Autodesk Inventor part; units mm, degrees
ref_plane "YZ Plane" through (0, 0, 0) normal (1, 0, 0) x (0, 1, 0)
ref_plane "XZ Plane" through (0, 0, 0) normal (0, 1, 0) x (-1, 0, 0)
ref_plane "XY Plane" through (0, 0, 0) normal (0, 0, 1) x (1, 0, 0)
sketch "スケッチ1" plane through (0, 0, 0) normal (0, 0, 1) x (1, 0, 0)
  line L0 (-9.75, -19.5) -> (9.75, -19.5) construction
  line L1 (9.75, -19.5) -> (9.75, 19.5) construction
  line L2 (9.75, 19.5) -> (-9.75, 19.5) construction
  line L3 (-9.75, 19.5) -> (-9.75, -19.5) construction
  line L4 (-9.75, -19.5) -> (9.75, 19.5) construction
  line L5 (9.75, -19.5) -> (-9.75, 19.5) construction
  line L6 (-9.75, 10.5) -> (-9.75, 19.5) construction
  line L7 (-9.75, 19.5) -> (9.75, 19.5)
  line L8 (9.75, 19.5) -> (9.75, 10.5) construction
  line L9 (-9.75, 10.5) -> (-11.75, 10.5)
  line L10 (-11.75, 10.5) -> (-11.75, -10.5)
  line L11 (-11.75, -10.5) -> (-9.75, -10.5)
  line L12 (-9.75, -10.5) -> (-9.75, -19.5) construction
  line L13 (-9.75, -19.5) -> (9.75, -19.5)
  line L14 (9.75, -19.5) -> (9.75, -10.5) construction
  line L15 (9.75, -10.5) -> (12.75, -10.5)
  line L16 (12.75, -10.5) -> (12.75, 10.5)
  line L17 (12.75, 10.5) -> (9.75, 10.5)
  line L18 (0, 0) -> (12.75, 0) construction
  circle A0 centre (-9.75, 11.55) radius 1.05 construction
  circle A1 centre (-9.75, -11.55) radius 1.05 construction
  circle A2 centre (9.75, 11.55) radius 1.05 construction
  circle A3 centre (9.75, -11.55) radius 1.05 construction
  line L19 (-9.75, 19.5) -> (-9.75, 12.6)
  arc A4 (-9.75, 10.5) -> (-9.75, 12.6) centre (-9.75, 11.55) ccw
  arc A5 (-9.75, -12.6) -> (-9.75, -10.5) centre (-9.75, -11.55) ccw
  line L20 (-9.75, -12.6) -> (-9.75, -19.5)
  line L21 (9.75, 12.6) -> (9.75, 19.5)
  arc A6 (9.75, 12.6) -> (9.75, 10.5) centre (9.75, 11.55) ccw
  line L22 (9.75, -12.6) -> (9.75, -19.5)
  arc A7 (9.75, -10.5) -> (9.75, -12.6) centre (9.75, -11.55) ccw
  dimension "d21" = 2
  dimension "d23" = 3
  dimension "d30" = 19.5
  dimension "d48" = 9
  dimension "d49" = 39
  dimension "d50" = 2.1
extrude "押し出し1" add sketch "スケッチ1" along normal blind 5
sketch "スケッチ2" plane through (9.75, -19.5, 0) normal (1, 0, 0) x (0, 0, -1)
  line L0 (0, 0) -> (-5, 0)
  line L1 (0, 39) -> (-5, 39)
  point P0 (0, 19.5)
  point P1 (-2.5, 4)
  point P2 (-2.5, 35)
  point P3 (-2.5, 0)
  dimension "d53" = 4
  dimension "d54" = 4
hole "穴1" at (9.75, -15.5, 2.5) at (9.75, 15.5, 2.5) direction (-1, 0, 0) diameter 2.459 depth 2.5 tip angle 118
mirror "ミラー1" about plane through (0, 0, 0) normal (1, 0, 0) of "穴1"
sketch "スケッチ3" plane through (0, 0, 5) normal (0, 0, 1) x (1, 0, 0)
  line L0 (9.75, 12.6) -> (9.75, 19.5)
  line L1 (-9.75, 19.5) -> (-9.75, 12.6)
  line L2 (-14.3307, 15.6684) -> (-9.75, 15.6684)
  line L3 (-9.75, 15.6684) -> (-9.75, -16.7148)
  line L4 (-9.75, -16.7148) -> (-14.3307, -16.7148)
  line L5 (-14.3307, -16.7148) -> (-14.3307, 15.6684)
  line L6 (15.2214, 11.55) -> (9.75, 11.55)
  line L7 (9.75, 11.55) -> (9.75, -15.9078)
  line L8 (9.75, -15.9078) -> (15.2214, -15.9078)
  line L9 (15.2214, -15.9078) -> (15.2214, 11.55)
  point P0 (0, 0)
extrude "押し出し2" cut sketch "スケッチ3" against normal blind 2.5
sketch "スケッチ4" plane through (0, 0, 5) normal (0, 0, 1) x (1, 0, 0)
  line L0 (9.75, 12.6) -> (9.75, 19.5)
  line L1 (9.75, 19.5) -> (-9.75, 19.5)
  line L2 (-9.75, -12.6) -> (-9.75, -19.5)
  line L3 (-9.75, -19.5) -> (9.75, -19.5)
  line L4 (-5.75, 15.5) -> (5.75, 15.5) construction
  line L5 (5.75, 15.5) -> (5.75, -15.5) construction
  line L6 (5.75, -15.5) -> (-5.75, -15.5) construction
  line L7 (-5.75, -15.5) -> (-5.75, 15.5) construction
  line L8 (5.75, 15.5) -> (-5.75, -15.5) construction
  line L9 (3.6168, 15.5) -> (-5.75, 15.5)
  line L10 (-5.75, 15.5) -> (-5.75, -9.7497)
  line L11 (-5.75, -9.7497) -> (3.6168, 15.5)
  line L12 (-3.6168, -15.5) -> (5.75, -15.5)
  line L13 (5.75, -15.5) -> (5.75, 9.7497)
  line L14 (5.75, 9.7497) -> (-3.6168, -15.5)
  point P0 (0, 0)
  dimension "d64" = 4
  dimension "d65" = 4
  dimension "d66" = 4
  dimension "d67" = 4
  dimension "d68" = 4
extrude "押し出し3" cut sketch "スケッチ4" against normal blind 5
fillet "フィレット1" radius 1.05 6 edges at (-3.6168, -15.5, 2.5) (-5.75, 15.5, 2.5) (3.6168, 15.5, 2.5) (5.75, 9.7497, 2.5) (-5.75, -9.7497, 2.5) (5.75, -15.5, 2.5)
equation "\"d48\" = d26 + d35"
equation "\"d49\" = d38"
equation "\"d66\" = d65"
equation "\"d68\" = d67"
properties part number "胴体_メインフレーム_1_12" material "アセタール樹脂、黒"
The model under review builds one solid part; all positions refer to its coordinate system, in mm. A direction names the side the tool comes from. Give positions to 0.01 mm unless a question says otherwise; leave off trailing zeros. Order: outer loops, then holes, each group sorted by start corner. A loop starts at its lowest first (then second) coordinate and runs counter-clockwise, first axis right, second up. Notation, with made-up numbers: (10, 16.5) - (15, 16.5) arc R23 cw to (15, 31.5) - close; hole circle Ø5 at (63.25, 3). An arc over 180 degrees is marked (long way). Use CSV: the item, a comma, the result in double quotes. Start each with the question number.
Q1. Tool access review of faces 5 (the cylindrical face through (-8.48, -14.28, 2.66)), 6 (the cylindrical face through (8.48, -16.72, 2.66)), 7 (the flat face through (11, 10.5, 1)), 8 (the flat face through (-9.75, 17, 2)), 9 (the flat face through (-1, 15.5, 3)): name each direction out of +Z, -Z, +X, -X, +Y, -Y from which nothing blocks a thin tool from reaching the whole face with its end or side.
Q2. We need section C-C, the plane x = 9.25. Write out the cut boundary in (y, z).
Q3. We need section B-B, the plane y = 6. Write out the cut boundary in (x, z), and give its area (3 significant figures).
Q4. We need section D-D, the plane y = -1.5. Write out the cut boundary in (x, z).
Q5. Clearance check with flat-ended pins moving along their axes: pin 1 Ø0.8 at (x, z) = (11, 1) entering from +Y; pin 2 Ø1.2 at (y, z) = (-0.5, 4) entering from +X; pin 3 Ø1.6 at (x, y) = (-11, 4.5) entering from +Z. State where each tip first meets the part, or that it passes through.
Q6. The part is to be moulded in two halves that separate along X. For faces 1 (the conical face through (-6.64, -15.71, 2.53)), 2 (the cylindrical face through (-4.865, -4.937, 2.465)), 3 (the cylindrical face through (-5.451, 15.184, 2.465)), 4 (the flat face through (0, 19.5, 2)), say which applies: +X half, -X half, draft (parallel to the pull), parting line (faces both ways), or undercut.
Q7. To check wall thickness, follow line 1 along Y through (x, z) = (-8.05, 2.5); line 2 along Y through (x, z) = (-8.85, 2.5); line 3 along Y through (x, z) = (-9.15, 2.5). State the ranges of each line that lie inside material, in increasing order. Write a range as [from, to].
Q8. We need section A-A, the plane z = 0.45. Write out the cut boundary in (x, y), and give its area (3 significant figures).
Outcome:
1,face 5,"-X"
1,face 6,"+X"
1,face 7,"+Z, -Z, +X, +Y"
1,face 8,"+Z, -Z, -X, +Y"
1,face 9,"+Z, -Z"
2,outline,"(-19.5, 0) - (-12.47, 0) - (-12.47, 5) - (-19.5, 5) - close; (-10.63, 0) - (10.63, 0) - (10.63, 5) - (-10.63, 5) - close; (12.47, 0) - (19.5, 0) - (19.5, 5) - (12.47, 5) - close; hole circle Ø2.46 at (-15.5, 2.5); hole circle Ø2.46 at (15.5, 2.5)"
3,outline,"(-11.75, 0) - (-5.75, 0) - (-5.75, 5) - (-9.75, 5) - (-9.75, 2.5) - (-11.75, 2.5) - close; (0.09, 0) - (12.75, 0) - (12.75, 2.5) - (9.75, 2.5) - (9.75, 5) - (0.09, 5) - close"
3,area,"80.8 mm^2"
4,outline,"(-11.75, 0) - (-5.75, 0) - (-5.75, 5) - (-9.75, 5) - (-9.75, 2.5) - (-11.75, 2.5) - close; (-2.69, 0) - (1.58, 0) - (1.58, 5) - (-2.69, 5) - close; (5.75, 0) - (12.75, 0) - (12.75, 2.5) - (9.75, 2.5) - (9.75, 5) - (5.75, 5) - close"
5,pin 1,"stops at y = 10.5"
5,pin 2,"stops at x = 9.75"
5,pin 3,"stops at z = 2.5"
6,face 1,"-X half"
6,face 2,"undercut"
6,face 3,"undercut"
6,face 4,"draft"
7,line 1,"y = [-19.5, -16.73], [-14.27, 14.27], [16.73, 19.5]"
7,line 2,"y = [-19.5, -16.73], [-14.27, -12.09], [-11.01, 11.01], [12.09, 14.27], [16.73, 19.5]"
7,line 3,"y = [-19.5, -16.73], [-14.27, -12.41], [-10.69, 10.69], [12.41, 14.27], [16.73, 19.5]"
8,outline,"(-11.75, -10.5) - (-9.75, -10.5) arc R1.05 cw to (-9.75, -12.6) - (-9.75, -19.5) - (9.75, -19.5) - (9.75, -12.6) arc R1.05 cw to (9.75, -10.5) - (12.75, -10.5) - (12.75, 10.5) - (9.75, 10.5) arc R1.05 cw to (9.75, 12.6) - (9.75, 19.5) - (-9.75, 19.5) - (-9.75, 12.6) arc R1.05 cw to (-9.75, 10.5) - (-11.75, 10.5) - close; hole (-5.75, -3.9) arc R1.05 ccw to (-3.72, -4.27) - (3.09, 14.08) arc R1.05 ccw to (2.11, 15.5) - (-4.7, 15.5) arc R1.05 ccw to (-5.75, 14.45) - close; hole (-3.09, -14.08) arc R1.05 ccw to (-2.11, -15.5) - (4.7, -15.5) arc R1.05 ccw to (5.75, -14.45) - (5.75, 3.9) arc R1.05 ccw to (3.72, 4.27) - close"
8,area,"633 mm^2"
